Part model, mm, in its own coordinate system. A direction names the side the tool comes from. Coordinates: 2 decimals unless noted, no trailing zeros. Order: outer loops, then holes, each group sorted by start corner. A loop starts at its lowest first (then second) coordinate and runs counter-clockwise, first axis right, second up.
1) Mould opens along X. For faces 6 (the flat face through (8.104, 4, 0)), 7 (the cylindrical face through (-9.048, 0.977, 0.903)), 8 (the flat face through (-2.945, 2.5, 0.1)) say: +X half, -X half, draft (parallel to the pull), parting line (faces both ways), or undercut.
2) Cut at A-A (z = -0.5). List the corners of the cut face in (x, y), and give its area (3 significant figures).
3) Tool access for faces 1 (the flat face through (4, 8.485, 0)), 2 (the flat face through (0, 2.984, 0)), 3 (the flat face through (-1, 2, 3.882)), 4 (the flat face through (-2.945, -0.5, 0.1)), 5 (the flat face through (3, -1.003, 0)): list every direction of +Z, -Z, +X, -X, +Y, -Y with a clear straight run to the whole face (end or side of a thin tool).
4) Cut at D-D (y = 2.75). List the corners of the cut face in (x, z).
5) Cut at C-C (x = -11). List the corners of the cut face in (y, z).
6) Cut at B-B (z = 2.75). List the corners of the cut face in (x, y).
7) Pin check, flat tips, straight feed: pin 1 Ø4 at (x, z) = (-10, 0) entering from +Y; pin 2 Ø0.5 at (y, z) = (-0.5, -1) entering from -X; pin 3 Ø4 at (x, z) = (-10, 1) entering from -Y. Stop position of each tip, or through.
8) Wall check: L1, parallel to Y at x = 3.5, z = -2.75; L2, parallel to X at y = 7, z = 3; L3, parallel to Y at x = -2, z = -2.5. Give the ranges that are in metal, low to high.
Autodesk Inventor part; units mm, degrees
ref_plane "YZ Plane" through (0, 0, 0) normal (1, 0, 0) x (0, 1, 0)
ref_plane "XZ Plane" through (0, 0, 0) normal (0, 1, 0) x (-1, 0, 0)
ref_plane "XY Plane" through (0, 0, 0) normal (0, 0, 1) x (1, 0, 0)
sketch "Sketch1" plane through (0, 0, 0) normal (0, 1, 0) x (-1, 0, 0)
  line L0 (15.6447, 3.8822) -> (-8.1043, 3.8822)
  line L1 (-8.1043, 3.8822) -> (-8.1043, -3.7378)
  line L2 (-8.1043, -3.7378) -> (15.6447, -3.7378)
  line L3 (15.6447, -3.7378) -> (15.6447, 3.8822)
  point P0 (0, 0)
  dimension "d0" = 23.749
  dimension "d1" = 7.62
extrude "Extrusion1" add sketch "Sketch1" along normal blind 1.9812
sketch "Sketch2" plane through (8.1043, 0, 3.8822) normal (1, 0, 0) x (0, 0, -1)
  line L0 (0, 0) -> (0, 1.9812)
  line L1 (0, 0.9906) -> (0, 2.9845)
  line L2 (0, 2.9845) -> (7.62, 2.9845)
  line L3 (7.62, 2.9845) -> (7.62, -1.0033)
  line L4 (7.62, -1.0033) -> (0, -1.0033)
  line L5 (0, -1.0033) -> (0, 2.9845)
  point P0 (3.8822, 0)
  dimension "d4" = 1.9939
  dimension "d5" = 3.9878
extrude "Extrusion2" add sketch "Sketch2" against normal blind 11.049
sketch "Sketch3" plane through (8.1043, 2.9845, 3.8822) normal (0, 1, 0) x (1, 0, 0)
  line L0 (0, 0) -> (0, 7.62)
  line L1 (0, 7.62) -> (-11.049, 7.62)
  line L2 (0, 0) -> (-5.08, 0)
  line L3 (-5.08, 0) -> (-5.08, 7.62)
  line L4 (-5.08, 7.62) -> (0, 7.62)
  line L5 (0, 7.62) -> (0, 0)
  point P0 (-8.1043, 3.8822)
  dimension "d8" = 5.08
extrude "Extrusion3" add sketch "Sketch3" along normal blind 5.9944
sketch "Sketch4" plane through (-15.6447, 0, 3.8822) normal (0, 0, 1) x (1, 0, 0)
  line L0 (18.669, 2.9845) -> (18.669, 8.9789)
  line L1 (18.669, 8.9789) -> (18.669, 6.9849)
  line L2 (18.669, 6.9849) -> (21.21, 6.9849)
  circle A0 centre (21.21, 6.9849) radius 1.5
  line L3 (21.21, 8.4849) -> (18.669, 8.4849)
  line L4 (21.21, 5.4849) -> (18.669, 5.4849)
  line L5 (18.669, 8.4849) -> (18.669, 5.4849)
  point P0 (15.6447, 0)
  dimension "d11" = 1.994
  dimension "d12" = 2.541
  dimension "d13" = 3
extrude "Extrusion4" cut sketch "Sketch4" against normal blind 10
sketch "Sketch5" plane through (0, 1.9812, 0) normal (0, 1, 0) x (1, 0, 0)
  line L0 (-15.6447, 3.7378) -> (-15.6447, -3.8822)
  line L1 (-15.6447, -0.0722) -> (-10.6447, -0.0722)
  point P0 (0, 0)
  dimension "d16" = 5
hole "Hole1" at (-10.6447, 1.9812, 0.0722) direction (0, -1, 0) diameter 3.6 end through all
properties part number "end axle"
Geometry check:
1. face 6: +X half
1. face 7: undercut
1. face 8: -X half
2. outline: (-15.64, 0) - (-12.35, 0) - (-12.35, 1.98) - (-15.64, 1.98) - close; (-8.94, 0) - (-2.94, 0) - (-2.94, -1) - (8.1, -1) - (8.1, 8.98) - (3.02, 8.98) - (3.02, 8.48) - (5.57, 8.48) arc R1.5 cw to (5.57, 5.48) - (3.02, 5.48) - (3.02, 2.98) - (-2.94, 2.98) - (-2.94, 1.98) - (-8.94, 1.98) - close
2. area: 81.8 mm2
3. face 1: +Z, -Z, -X
3. face 2: +Z, -Z, -X, +Y
3. face 3: +Z, +X, -X, +Y, -Y
3. face 4: +Z, -Z, -X, -Y
3. face 5: +Z, -Z, +X, -X, -Y
4. outline: (-2.94, -3.74) - (8.1, -3.74) - (8.1, 3.88) - (-2.94, 3.88) - close
5. outline: (0, -3.74) - (1.98, -3.74) - (1.98, -1.69) - (0, -1.69) - close; (0, 1.84) - (1.98, 1.84) - (1.98, 3.88) - (0, 3.88) - close
6. outline: (-15.64, 0) - (-2.94, 0) - (-2.94, -1) - (8.1, -1) - (8.1, 8.98) - (3.02, 8.98) - (3.02, 8.48) - (5.57, 8.48) arc R1.5 cw to (5.57, 5.48) - (3.02, 5.48) - (3.02, 2.98) - (-2.94, 2.98) - (-2.94, 1.98) - (-15.64, 1.98) - close
7. pin 1: stops at y = 1.98
7. pin 2: stops at x = -2.94
7. pin 3: stops at y = 0
8. L1: y = -1 to 5.48, 8.48 to 8.98
8. L2: x = 7.07 to 8.1
8. L3: y = -1 to 2.98
